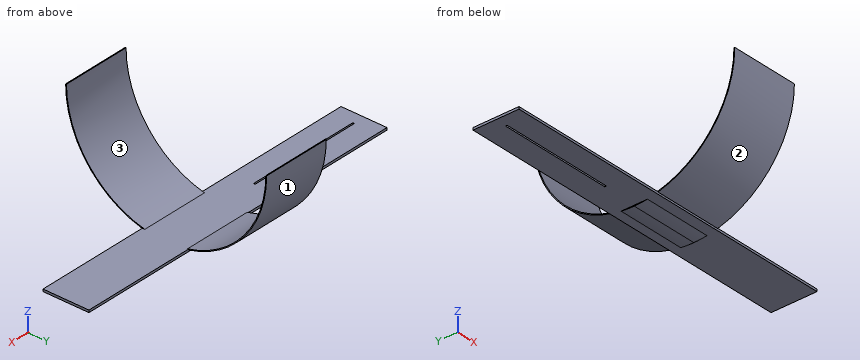
from build123d import *

# Parameters (mm, degrees)
SZKIC4_W                    = 150
SZKIC4_H                    = 20
SZKIC4_W_2                  = 50
SZKIC4_H_2                  = 0.7
DODANIE_WYCI_GNI_CIE1_DEPTH = 1
DODANIE_WYCI_GNI_CIE2_DEPTH = 30


with BuildPart() as part:
    # Szkic4 → Dodanie-wyciągnięcie1 (new body)
    with BuildSketch(Plane.XY):
        with Locations((44.938160122, 0.128489408)):
            Rectangle(SZKIC4_W, SZKIC4_H)
        Rectangle(SZKIC4_W_2, SZKIC4_H_2, mode=Mode.SUBTRACT)
    extrude(amount=DODANIE_WYCI_GNI_CIE1_DEPTH)

    # Szkic8 → Dodanie-wyciągnięcie2 (add)
    with BuildSketch(Plane(origin=(69.938160122, 0, 0), x_dir=(0, 0, -1), z_dir=(1, 0, 0))):
        with BuildLine():
            ThreePointArc((0.375817697, 0.480392187), (-12.438260626, 31.416313864), (-43.374182303, 44.230392187))
            Line((-43.374182303, 44.230392187), (-43.374182303, 43.857234708))
            ThreePointArc((-43.374182303, 43.857234708), (-12.70212281, 31.15245168), (0.002660218, 0.480392187))
            ThreePointArc((0.002660218, 0.480392187), (-12.70212281, -30.191667306), (-43.374182303, -42.896450334))
            Line((-43.374182303, -42.896450334), (-43.374182303, -43.269607813))
            ThreePointArc((-43.374182303, -43.269607813), (-12.438260626, -30.45552949), (0.375817697, 0.480392187))
        make_face()
    extrude(amount=-DODANIE_WYCI_GNI_CIE2_DEPTH)


solid = part.part
The listing builds one solid part. Answer for the finished solid, in the listing's coordinates (mm). Face numbers are marked on the shaded views. Give positions to 0.01 mm unless a question says otherwise; leave off trailing zeros. Loops run counter-clockwise (first coordinate to the right, second up) from the corner with the lowest first, then second, coordinate; pieces in that order, holes last. Notation, with made-up numbers: (-4, 30) - (51, 30) arc R29 cw to (51, 58) - close; hole circle Ø8 at (57, -18.75). An arc over 180 degrees is marked (long way). Use one line per item in the form item = value.
1. The mould has two halves that part along Y. Classify the marked faces 1, 2 and 3: pulls with the +Y half, pulls with the -Y half, needs draft (parallel to the pull), parting line crosses it, or undercut.
Calculated:
face_1 = pulls with the +Y half
face_2 = pulls with the -Y half
face_3 = undercut
2. Section B-B on z = 22.5 is taken. Give the vertices of the cut face in (x, y).
Calculated:
outline = (39.94, -37.97) - (69.94, -37.97) - (69.94, -37.54) - (39.94, -37.54) - close; (39.94, 38.5) - (69.94, 38.5) - (69.94, 38.93) - (39.94, 38.93) - close
3. Find the intervals of material crossed by line 1 along Y through (x, z) = (65, 12); line 2 along Z through (x, y) = (-20, 6); line 3 along Y through (x, z) = (66, 34.5), in increasing order. Write a range as [from, to].
Calculated:
line_1 = [-30.01, -29.47], [30.43, 30.97]
line_2 = [0, 1]
line_3 = [-42.36, -41.98], [42.94, 43.32]
4. Section D-D on y = 4.5 is taken. Give the vertices of the cut face in (x, z).
Calculated:
outline = (-30.06, 0) - (39.94, 0) - (39.94, -0.19) - (69.94, -0.19) - (69.94, 0) - (119.94, 0) - (119.94, 1) - (-30.06, 1) - close
5. Given pin 1 Ø1.1 at (x, z) = (27.5, 0.5) entering from +Y; pin 2 Ø10 at (x, y) = (74, -4.5) entering from +Z; pin 3 Ø17 at (y, z) = (-31.5, 20.5) entering from +X; pin 4 Ø22 at (x, y) = (76, -3.5) entering from -Z, each flat-ended and moving along its own axis, determine where each tip first touches the part or whether it passes through.
Calculated:
pin_1 = 10.13
pin_2 = 1
pin_3 = 69.94
pin_4 = -0.38
6. Section A-A on x = 12 is taken. Give the vertices of the cut face in (y, z), then the cut area to 3 significant figures.
Calculated:
outline = (-9.87, 0) - (-0.35, 0) - (-0.35, 1) - (-9.87, 1) - close; (0.35, 0) - (10.13, 0) - (10.13, 1) - (0.35, 1) - close
area = 19.3 mm^2
